Geometry: see drawing. Coordinates: mm, zero at the bounding-box minimum. A direction names the side the tool comes from. Round coordinates to 2 decimals unless told otherwise and drop trailing zeros. Loops run counter-clockwise (first coordinate to the right, second up) from the corner with the lowest first, then second, coordinate; pieces in that order, holes last.
(1) First-contact query: pin 1 Ø12 at (x, z) = (157, 17) entering from -Y; pin 2 Ø10 at (x, y) = (144.5, 13.5) entering from -Z; pin 3 Ø15 at (x, y) = (173.5, 64.5) entering from -Z. Flat tips, straight axial feed; report the tip coordinate or a pass-through.
(2) Section B-B, the plane x = 131.5. Return the cut outline in (y, z).
(3) Material intervals for probe 1 along X at (y, z) = (34.5, 93) (1 decimal); probe 2 along X at (y, z) = (85, 48); probe 3 along Z at (x, y) = (194, 41.5), sorted ascending.
(4) Section A-A, the plane y = 54.5. Return the cut outline in (x, z).
(5) Section C-C, the plane y = 19. Return the cut outline in (x, z) (1 decimal).
(6) Section D-D, the plane x = 168. Return the cut outline in (y, z) (1 decimal), plus the area to 3 significant figures.
(7) Mould query, pull axis X, two halves, no side actions, for the marked faces 5, 6, 7 and 8. Classes: pulls with the +X half, pulls with the -X half, needs draft (parallel to the pull), parting line crosses it, or undercut.
(8) Set-up query: the marked faces 1, 2, 3 and 4. Return all of +Z, -Z, +X, -X, +Y, -Y with unobstructed straight access to the full face (end or side cutting, diameter ignored); none if empty.
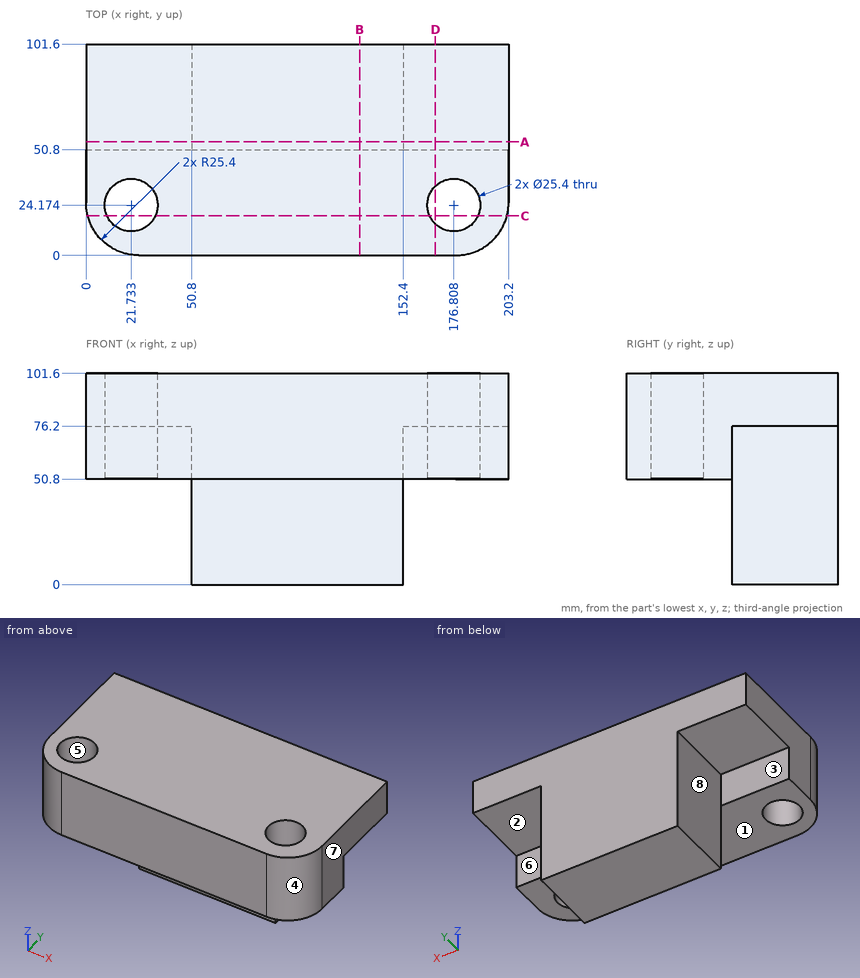
Output values:
1. pin 1: stops at y = 50.8
1. pin 2: stops at z = 50.8
1. pin 3: stops at z = 76.2
2. outline: (0, 50.8) - (50.8, 50.8) - (50.8, 0) - (101.6, 0) - (101.6, 101.6) - (0, 101.6) - close
3. probe 1: x = 0 to 14.3, 29.1 to 169.4, 184.2 to 203.2
3. probe 2: x = 50.8 to 152.4
3. probe 3: z = 50.8 to 101.6
4. outline: (0, 76.2) - (50.8, 76.2) - (50.8, 0) - (152.4, 0) - (152.4, 76.2) - (203.2, 76.2) - (203.2, 101.6) - (0, 101.6) - close
5. outline: (0.8, 50.8) - (10.1, 50.8) - (10.1, 101.6) - (0.8, 101.6) - close; (33.3, 50.8) - (165.2, 50.8) - (165.2, 101.6) - (33.3, 101.6) - close; (188.4, 50.8) - (202.4, 50.8) - (202.4, 101.6) - (188.4, 101.6) - close
6. outline: (0, 50.8) - (15, 50.8) - (15, 101.6) - (0, 101.6) - close; (33.3, 50.8) - (50.8, 50.8) - (50.8, 76.2) - (101.6, 76.2) - (101.6, 101.6) - (33.3, 101.6) - close
6. area: 2,940 mm2
7. face 5: undercut
7. face 6: needs draft
7. face 7: pulls with the +X half
7. face 8: pulls with the -X half
8. face 1: -Z, +X, -X, -Y
8. face 2: -Z, +X, +Y
8. face 3: -Z, -X, +Y
8. face 4: +Z, -Z, +X, -Y
